Source: CAD feature listing. Evaluate the final solid. Frame: model axes, mm. Face numbers are marked on the shaded views. A direction names the side the tool comes from. Round coordinates to 2 decimals unless told otherwise and drop trailing zeros. Order: outer loops, then holes, each group sorted by start corner. A loop starts at its lowest first (then second) coordinate and runs counter-clockwise, first axis right, second up. Notation, with made-up numbers: (38, 35) -> (84, 35) arc R18 ccw to (84, 49) -> close; hole circle Ø11 at (76.25, -27). An arc over 180 degrees is marked (long way). Answer as CSV lines item,"result".
from build123d import *

# Parameters (mm, degrees)
CROQUIS1_W              = 28
CROQUIS1_H              = 28
CROQUIS1_R              = 8.05
SALIENTE_EXTRUIR1_DEPTH = 3.25
CROQUIS2_W              = 28
CROQUIS2_H              = 28
CROQUIS2_R              = 8.6
SALIENTE_EXTRUIR2_DEPTH = 6
CORTAR_EXTRUIR1_DEPTH   = 3.5
CROQUIS6_R              = 1.5
CORTAR_EXTRUIR2_DEPTH   = 23.5
CROQUIS7_W              = 2.5
CROQUIS7_H              = 5
CROQUIS7_W_2            = 10
CROQUIS7_H_2            = 4
SALIENTE_EXTRUIR3_DEPTH = 3
REDONDEO1_R             = 5


with BuildPart() as part:
    # Croquis1 → Saliente-Extruir1 (new, symmetric)
    with BuildSketch(Plane.XY):
        Rectangle(CROQUIS1_W, CROQUIS1_H)
        with Locations(Location((0, 0, 0), (0, 0, 180))):
            Circle(CROQUIS1_R, mode=Mode.SUBTRACT)
    extrude(amount=SALIENTE_EXTRUIR1_DEPTH, both=True)

    # Croquis2 → Saliente-Extruir2 (add)
    with BuildSketch(Plane.XY.offset(3.25)):
        Rectangle(CROQUIS2_W, CROQUIS2_H)
        Circle(CROQUIS2_R, mode=Mode.SUBTRACT)
    extrude(amount=SALIENTE_EXTRUIR2_DEPTH)

    # Croquis3 → Cortar-Extruir1 (cut)
    with BuildSketch(Plane.XY.offset(9.25)):
        Polygon((11.029978213, 12.15), (7.970021787, 12.15), (6.440043573, 9.5), (7.970021787, 6.85), (11.029978213, 6.85), (12.559956427, 9.5), align=None)
        Polygon((-6.440043573, 9.5), (-7.970021787, 12.15), (-11.029978213, 12.15), (-12.559956427, 9.5), (-11.029978213, 6.85), (-7.970021787, 6.85), align=None)
        Polygon((-7.970021787, -6.85), (-11.029978213, -6.85), (-12.559956427, -9.5), (-11.029978213, -12.15), (-7.970021787, -12.15), (-6.440043573, -9.5), align=None)
        Polygon((11.029978213, -6.85), (7.970021787, -6.85), (6.440043573, -9.5), (7.970021787, -12.15), (11.029978213, -12.15), (12.559956427, -9.5), align=None)
    extrude(amount=-CORTAR_EXTRUIR1_DEPTH, mode=Mode.SUBTRACT)

    # Croquis6 → Cortar-Extruir2 (cut)
    with BuildSketch(Plane(origin=(0, 0, -3.25), x_dir=(-1, 0, 0), z_dir=(0, 0, -1))):
        with Locations((-9.5, 9.5)):
            Circle(CROQUIS6_R)
        with Locations((9.5, 9.5)):
            Circle(CROQUIS6_R)
        with Locations((9.5, -9.5)):
            Circle(CROQUIS6_R)
        with Locations((-9.5, -9.5)):
            Circle(CROQUIS6_R)
    extrude(amount=-CORTAR_EXTRUIR2_DEPTH, mode=Mode.SUBTRACT)

    # Croquis7 → Saliente-Extruir3 (add)
    with BuildSketch(Plane(origin=(0, 0, -3.25), x_dir=(-1, 0, 0), z_dir=(0, 0, -1))):
        Polygon((14, 5.5), (14, 2.5), (16.5, 2.5), (18.9, 2.5), (18.9, 5.5), align=None)
        with Locations((15.25, 0)):
            Rectangle(CROQUIS7_W, CROQUIS7_H)
        Polygon((14, -2.5), (14, -5.5), (18.9, -5.5), (18.9, -2.5), (16.5, -2.5), align=None)
        with Locations((0, -16)):
            Rectangle(CROQUIS7_W_2, CROQUIS7_H_2)
        with Locations((-15.25, 0)):
            Rectangle(CROQUIS7_W, CROQUIS7_H)
    extrude(amount=-SALIENTE_EXTRUIR3_DEPTH)

    # Redondeo1
    redondeo1_edges = [part.edges().sort_by_distance(p)[0] for p in [
        (14, -14, 3),
        (-14, -14, 3),
        (-14, 14, 3),
        (14, 14, 3),
    ]]
    fillet(redondeo1_edges, radius=REDONDEO1_R)


solid = part.part
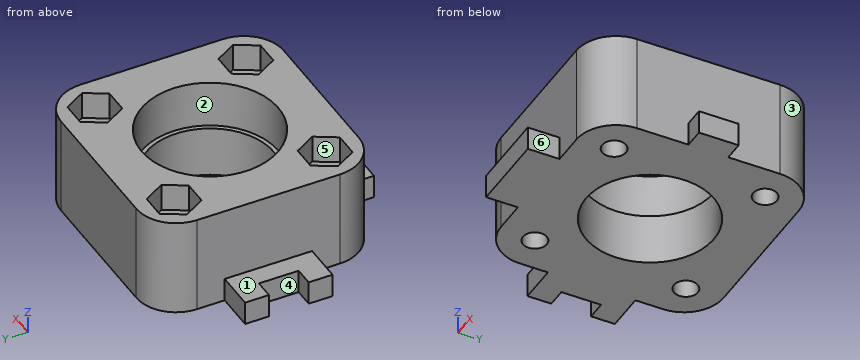
1. Section query C-C on x = 0. Return loops of the section in (y, z), and give its area (3 significant figures).
Results below:
outline,"(-18, -3.25) -> (-8.05, -3.25) -> (-8.05, 3.25) -> (-8.6, 3.25) -> (-8.6, 9.25) -> (-14, 9.25) -> (-14, -0.25) -> (-18, -0.25) -> close; (8.05, -3.25) -> (14, -3.25) -> (14, 9.25) -> (8.6, 9.25) -> (8.6, 3.25) -> (8.05, 3.25) -> close"
area,"154 mm2"
2. Pin query (flat end, axial travel): pin 1 (2.5 mm diameter, centred on x = 9.5, z = 7, fed in from +Y); pin 2 (0.9 mm diameter, centred on x = 9.5, z = 8, fed in from -Y); pin 3 (2.5 mm diameter, centred on x = -9.5, y = -10.5, fed in from +Z); pin 4 (2 mm diameter, centred on x = 0.5, y = -16, fed in from +Z). Return the tip coordinate at first contact, or that it passes through.
Results below:
pin 1,"y = 14"
pin 2,"y = -14"
pin 3,"z = 5.75"
pin 4,"z = -0.25"
3. Line query: L1, parallel to Y at x = -9.5, z = -0.5; L2, parallel to Y at x = 12.5, z = 6.25; L3, parallel to Y at x = 2, z = 5.5. Output: solid intervals per line, ascending. Write a range as [from, to].
Results below:
L1,"[-13.97, -11], [-8, 8], [11, 13.97]"
L2,"[-12.57, -9.6], [-9.4, 9.4], [9.6, 12.57]"
L3,"[-14, -8.36], [8.36, 14]"
4. Reachability of the marked faces 4, 5 and 6 from +Z, -Z, +X, -X, +Y, -Y: full face, straight path, thin tool, end or side. Return the list, or none.
Results below:
face 4,"+Z, -Z, -X"
face 5,"+Z"
face 6,"+Z, -Z, +X, -Y"
5. Section query A-A on y = 0. Return loops of the section in (x, z), and give its area (3 significant figures).
Results below:
outline,"(-16.5, -3.25) -> (-8.05, -3.25) -> (-8.05, 3.25) -> (-8.6, 3.25) -> (-8.6, 9.25) -> (-14, 9.25) -> (-14, -0.25) -> (-16.5, -0.25) -> close; (8.05, -3.25) -> (16.5, -3.25) -> (16.5, -0.25) -> (14, -0.25) -> (14, 9.25) -> (8.6, 9.25) -> (8.6, 3.25) -> (8.05, 3.25) -> close"
area,"157 mm2"
6. Section query D-D on x = 9.5. Return loops of the section in (y, z), and give its area (3 significant figures).
Results below:
outline,"(-13.97, -3.25) -> (-11, -3.25) -> (-11, 5.75) -> (-12.15, 5.75) -> (-12.15, 9.25) -> (-13.97, 9.25) -> close; (-8, -3.25) -> (8, -3.25) -> (8, 5.75) -> (6.85, 5.75) -> (6.85, 9.25) -> (-6.85, 9.25) -> (-6.85, 5.75) -> (-8, 5.75) -> close; (11, -3.25) -> (13.97, -3.25) -> (13.97, 9.25) -> (12.15, 9.25) -> (12.15, 5.75) -> (11, 5.75) -> close"
area,"258 mm2"
7. Section query B-B on z = 2.25. Return loops of the section in (x, y), and give its area (3 significant figures).
Results below:
outline,"(-14, -9) arc R5 ccw to (-9, -14) -> (9, -14) arc R5 ccw to (14, -9) -> (14, 9) arc R5 ccw to (9, 14) -> (-9, 14) arc R5 ccw to (-14, 9) -> close; hole circle Ø3 at (-9.5, -9.5); hole circle Ø3 at (-9.5, 9.5); hole circle Ø16.1 at (0, 0); hole circle Ø3 at (9.5, -9.5); hole circle Ø3 at (9.5, 9.5)"
area,"531 mm2"
8. Mould query, pull axis X, two halves, no side actions, for the marked faces 1, 2 and 3. Classes: released by +X, released by -X, zero draft, split by the parting line, or undercut.
Results below:
face 1,"zero draft"
face 2,"undercut"
face 3,"released by +X"
